from build123d import *

# Parameters (mm, degrees)
SKETCH1_W           = 42
SKETCH1_H           = 30
BOSS_EXTRUDE1_DEPTH = 15
FILLET1_R           = 5
CUT_EXTRUDE1_DEPTH  = 10.5
FILLET2_R           = 0.2
SKETCH3_R           = 3.5
BOSS_EXTRUDE2_DEPTH = 14.6
SKETCH4_R           = 5
BOSS_EXTRUDE3_DEPTH = 10.5
SKETCH5_R           = 3
CUT_EXTRUDE2_DEPTH  = 2
CUT_EXTRUDE2_DRAFT  = -47
SKETCH6_R           = 0.85526258
CUT_EXTRUDE3_DEPTH  = 39.078865697
SKETCH7_R           = 2.5
CUT_EXTRUDE4_DEPTH  = 30.849623234
BOSS_EXTRUDE4_DEPTH = 10.5
FILLET3_R           = 3
FILLET4_R           = 0.4
SKETCH9_R           = 11.5
CUT_EXTRUDE5_DEPTH  = 3


with BuildPart() as part:
    # Sketch1 → Boss-Extrude1 (new body)
    with BuildSketch(Plane(origin=(0, 0, 0), x_dir=(0, 0, -1), z_dir=(1, 0, 0))):
        Rectangle(SKETCH1_W, SKETCH1_H)
    extrude(amount=BOSS_EXTRUDE1_DEPTH)

    # Fillet1
    fillet1_edges = [part.edges().sort_by_distance(p)[0] for p in [
        (7.5, 15, 21),
        (7.5, 15, -21),
        (7.5, -15, 21),
    ]]
    fillet(fillet1_edges, radius=FILLET1_R)

    # Sketch2 → Cut-Extrude1 (cut)
    with BuildSketch(Plane(origin=(15, 0, 0), x_dir=(0, 0, -1), z_dir=(1, 0, 0))):
        with BuildLine():
            Line((21, 9), (11, 9))
            Line((11, 9), (11, 0.6))
            Line((11, 0.6), (6, 0.6))
            Line((6, 0.6), (6, 7))
            ThreePointArc((6, 7), (0, 13), (-6, 7))
            ThreePointArc((-6, 7), (-7.417424305, 10.872983346), (-11, 12.916079783))
            Line((-11, 12.916079783), (-11, 15))
            Line((-11, 15), (-12, 15))
            Line((-12, 15), (-12, 12))
            ThreePointArc((-12, 12), (-7.025319235, 7.50254481), (-11, 2.101020514))
            Line((-11, 2.101020514), (-7.7, -1.7))
            Line((-7.7, -1.7), (-4.7, -1.7))
            Line((-4.7, -1.7), (0, -5.6))
            Line((0, -5.6), (11, -5.6))
            Line((11, -5.6), (21, -5.6))
            Line((21, -5.6), (21, 9))
        make_face()
    extrude(amount=-CUT_EXTRUDE1_DEPTH, mode=Mode.SUBTRACT)

    # Fillet2
    fillet2_edges = [part.edges().sort_by_distance(p)[0] for p in [
        (9.75, 7, 6),
    ]]
    fillet(fillet2_edges, radius=FILLET2_R)

    # Sketch3 → Boss-Extrude2 (add)
    with BuildSketch(Plane(origin=(0, -5.6, 0), x_dir=(1, 0, 0), z_dir=(0, 1, 0))):
        with Locations(Location((10, 16, 0), (0, 0, 90))):
            Circle(SKETCH3_R)
    extrude(amount=BOSS_EXTRUDE2_DEPTH)

    # Sketch4 → Boss-Extrude3 (add)
    with BuildSketch(Plane(origin=(4.5, 0, 0), x_dir=(0, 0, -1), z_dir=(1, 0, 0))):
        with Locations(Location((0, 7, 0), (0, 0, 180))):
            Circle(SKETCH4_R)
    extrude(amount=BOSS_EXTRUDE3_DEPTH)


with BuildPart() as cut_extrude2_tool:
    # Sketch5 → Cut-Extrude2 (with draft: the straight prism first)
    with BuildSketch(Plane.XZ.offset(15)):
        with Locations((10, 6.5)):
            Circle(SKETCH5_R)
    extrude(amount=-CUT_EXTRUDE2_DEPTH)
    # Cut-Extrude2: the draft: its side faces are tilted about the plane it starts from
    cut_extrude2_sides = [cut_extrude2_tool.faces().sort_by_distance(p)[0] for p in [
        (7, -14, 6.5),
    ]]
    draft(cut_extrude2_sides, Plane.XZ.offset(15), CUT_EXTRUDE2_DRAFT)


with BuildPart() as part_1:
    add(part.part)

    # Cut-Extrude2: cut by cut_extrude2_tool
    add(cut_extrude2_tool.part, mode=Mode.SUBTRACT)

    # Sketch6 → Cut-Extrude3 (cut, through all)
    with BuildSketch(Plane.XZ.offset(13)):
        with Locations(Location((10, 6.5, 0), (0, 0, 270))):
            Circle(SKETCH6_R)
    extrude(amount=-CUT_EXTRUDE3_DEPTH, mode=Mode.SUBTRACT)

    # Sketch7 → Cut-Extrude4 (cut, through all)
    with BuildSketch(Plane(origin=(15, 0, 0), x_dir=(0, 0, -1), z_dir=(1, 0, 0))):
        with Locations((0, 7)):
            Circle(SKETCH7_R)
    extrude(amount=-CUT_EXTRUDE4_DEPTH, mode=Mode.SUBTRACT)

    # Sketch8 → Boss-Extrude4 (add)
    with BuildSketch(Plane(origin=(15, 0, 0), x_dir=(0, 0, -1), z_dir=(1, 0, 0))):
        with BuildLine():
            Line((21, -5.6), (24, -5.6))
            ThreePointArc((24, -5.6), (27.171714604, -5.939160103), (30.2, -6.941303137))
            Line((30.2, -6.941303137), (30.2, -8.9))
            ThreePointArc((30.2, -8.9), (25.6, -8.545235705), (21, -8.9))
            Line((21, -8.9), (21, -5.6))
        make_face()
    extrude(amount=-BOSS_EXTRUDE4_DEPTH)

    # Fillet3
    fillet3_edges = [part_1.edges().sort_by_distance(p)[0] for p in [
        (9.75, -8.9, -21),
        (7.5, -15, -21),
    ]]
    fillet(fillet3_edges, radius=FILLET3_R)

    # Fillet4
    fillet4_edges = [part_1.edges().sort_by_distance(p)[0] for p in [
        (9.75, -6.941303137, -30.2),
        (9.75, -8.9, -30.2),
    ]]
    fillet(fillet4_edges, radius=FILLET4_R)

    # Sketch9 → Cut-Extrude5 (cut)
    with BuildSketch(Plane.ZY):
        with Locations((0, 7)):
            Circle(SKETCH9_R)
    extrude(amount=-CUT_EXTRUDE5_DEPTH, mode=Mode.SUBTRACT)


solid = part_1.part
Geometry check sheet. Reference: the model listing, model coordinates, mm. A direction names the side the tool comes from. Round coordinates to 2 decimals unless told otherwise and drop trailing zeros. Loops run counter-clockwise (first coordinate to the right, second up) from the corner with the lowest first, then second, coordinate; pieces in that order, holes last.
Item 1: Cross-section at C-C on y = 4. Record the boundary of the cut face in (x, z), then the cut area to 3 significant figures.
Item 2: Cross-section at D-D on x = 10. Count the separate pieces of the cut face and the enclosed holes in it, then the cut area to 3 significant figures.
Item 3: Thickness scan on line 1 (Y direction, x = 6.5, z = 0); line 2 (Z direction, x = 10, y = 10.75); line 3 (Y direction, x = 3.5, z = 1.5). Record the ranges inside material, lowest first.
Item 4: Mould release check, pull along Z, two halves, no side actions. Record for faces 6 (the flat face through (15, 9, 2)), 7 (the flat face through (7, 0, 21)), 8 (the flat face through (10, 0.6, -9)), 9 (the flat face through (3, -1, -21)): pulls with the +Z half, pulls with the -Z half, needs draft (parallel to the pull), parting line crosses it, or undercut.
Item 5: Gauge pin test, flat ends, axial feed: pin 1 (6 mm diameter, centred on y = 0, z = 2.5, fed in from +X); pin 2 (4 mm diameter, centred on x = 10.5, y = 3.5, fed in from -Z); pin 3 (3 mm diameter, centred on y = -8.5, z = -27, fed in from -X); pin 4 (1.4 mm diameter, centred on x = 10, z = 6.5, fed in from -Y). Record the tip position at first contact, or that the pin passes through.
Item 6: Cross-section at A-A on y = -10.5. Record the boundary of the cut face in (x, z).
Item 7: Access from +Z, -Z, +X, -X, +Y, -Y to the whole of each face (thin tool, end or side, straight path). Record for faces 1 (the flat face through (6, 9, -16)), 2 (the flat face through (4.5, -7, -26)), 3 (the cylindrical face through (9.82, 11.39, 7.91)), 4 (the cylindrical face through (9.676, -9.558, -21.795)), 5 (the flat face through (3, 5, 2)).
Item 8: Cross-section at B-B on z = -10. Record the boundary of the cut face in (x, y).
Answer sheet:
1. outline: (0, -21) - (4.5, -21) - (4.5, -11) - (15, -11) - (15, -6) - (4.5, -6) - (4.5, -4) - (15, -4) - (15, 4) - (4.5, 4) - (4.5, 8) - (15, 8) - (15, 21) - (0, 21) - (0, 11.1) - (3, 11.1) - (3, -11.1) - (0, -11.1) - close; circle Ø7 at (10, -16)
1. area: 434 mm2
2. separate pieces: 4
2. enclosed holes: 1
2. area: 989 mm2
3. line 1: y = -15 to -5.6, 2 to 4.5, 9.5 to 12, 13 to 15
3. line 2: z = -20.94 to -4.68, -3.31 to 3.31, 4.68 to 5.64, 8.69 to 20.94
3. line 3: y = -15 to 5, 9 to 15
4. face 6: needs draft
4. face 7: pulls with the +Z half
4. face 8: undercut
4. face 9: pulls with the -Z half
5. pin 1: stops at x = 15
5. pin 2: stops at z = -19.5
5. pin 3: stops at x = 4.5
5. pin 4: passes through
6. outline: (0, -21) - (4.5, -21) - (4.5, -21.21) - (15, -21.21) - (15, 20.97) - (0, 20.97) - close; hole circle Ø1.71 at (10, 6.5)
7. face 1: none
7. face 2: -Z, -X, +Y, -Y
7. face 3: +X
7. face 4: +X, -X, -Y
7. face 5: -X
8. outline: (0, -15) - (15, -15) - (15, -5.6) - (4.5, -5.6) - (4.5, 0.6) - (15, 0.6) - (15, 15) - (0, 15) - (0, 12.68) - (3, 12.68) - (3, 1.32) - (0, 1.32) - close
